```python
from build123d import *

# Parameters (mm, degrees)
SKETCH1_R           = 10
SKETCH1_R_2         = 2
SKETCH1_R_3         = 1.5
BOSS_EXTRUDE1_DEPTH = 2.3
SKETCH2_R           = 2.915
CUT_EXTRUDE1_DEPTH  = 1


with BuildPart() as part:
    # Sketch1 → Boss-Extrude1 (new body)
    with BuildSketch(Plane(origin=(0, 16.875, 0), x_dir=(1, 0, 0), z_dir=(0, 1, 0))):
        Circle(SKETCH1_R)
        Circle(SKETCH1_R_2, mode=Mode.SUBTRACT)
        with Locations((0, 6)):
            Circle(SKETCH1_R_3, mode=Mode.SUBTRACT)
        with Locations((0, -6)):
            Circle(SKETCH1_R_3, mode=Mode.SUBTRACT)
    extrude(amount=BOSS_EXTRUDE1_DEPTH)

    # Sketch2 → Cut-Extrude1 (cut)
    with BuildSketch(Plane(origin=(0, 19.175, 0), x_dir=(1, 0, 0), z_dir=(0, 1, 0))):
        with Locations((0, 6)):
            Circle(SKETCH2_R)
        with Locations((0, -6)):
            Circle(SKETCH2_R)
    extrude(amount=-CUT_EXTRUDE1_DEPTH, mode=Mode.SUBTRACT)


solid = part.part
```
Input: part model. Units: mm. Frame: model coordinates. A direction names the side the tool comes from. Coordinates: 2 decimals unless noted, no trailing zeros. Write each loop counter-clockwise with the first axis right and the second up, starting at its lowest first coordinate (ties: lowest second). Pieces come first, ordered by that corner, then holes.
1) Section A-A on z = 6. Output: boundary loops of the cut face in (x, y) (3 decimals).
2) Section D-D on z = 0. Output: boundary loops of the cut face in (x, y) (3 decimals), and give its area (3 significant figures).
3) Set-up query: faces 1 (the cylindrical face through (-0.325, 17.516, -4.536)), 2 (the flat face through (1.3, 18.175, -4.7)). Return all of +Z, -Z, +X, -X, +Y, -Y with unobstructed straight access to the full face (end or side cutting, diameter ignored); none if empty.
4) Material intervals for line 1 along Z through (x, y) = (0, 17.3); line 2 along Z through (x, y) = (0, 18.55) (3 decimals); line 3 along X through (y, z) = (18.3, 0), sorted ascending.
5) Pin query (flat end, axial travel): pin 1 Ø1 at (y, z) = (18.5, -4.5) entering from -X; pin 2 Ø2.5 at (x, z) = (0, 0) entering from +Y; pin 3 Ø1.7 at (x, z) = (1, -6) entering from +Y (3 decimals); pin 4 Ø7.5 at (x, z) = (0, -6) entering from -Y (3 decimals). Return the tip coordinate at first contact, or that it passes through.
6) Section B-B on x = 0. Output: boundary loops of the cut face in (y, z) (3 decimals).
7) Mould query, pull axis X, two halves, no side actions, for faces 3 (the cylindrical face through (-2.17, 18.01, 9.76)), 4 (the flat face through (1.3, 18.175, 7.3)), 5 (the flat face through (-2.4, 16.875, -0.1)). Classes: pulls with the +X half, pulls with the -X half, needs draft (parallel to the pull), parting line crosses it, or undercut.
8) Section C-C on y = 17.4. Output: boundary loops of the cut face in (x, z), and give its area (3 significant figures).
Check result:
1. outline: (-8, 16.875) - (-1.5, 16.875) - (-1.5, 18.175) - (-2.915, 18.175) - (-2.915, 19.175) - (-8, 19.175) - close; (1.5, 16.875) - (8, 16.875) - (8, 19.175) - (2.915, 19.175) - (2.915, 18.175) - (1.5, 18.175) - close
2. outline: (-10, 16.875) - (-2, 16.875) - (-2, 19.175) - (-10, 19.175) - close; (2, 16.875) - (10, 16.875) - (10, 19.175) - (2, 19.175) - close
2. area: 36.8 mm2
3. face 1: +Y, -Y
3. face 2: +Y
4. line 1: z = -10 to -7.5, -4.5 to -2, 2 to 4.5, 7.5 to 10
4. line 2: z = -10 to -8.915, -3.085 to -2, 2 to 3.085, 8.915 to 10
4. line 3: x = -10 to -2, 2 to 10
5. pin 1: stops at x = -9.17
5. pin 2: passes through
5. pin 3: stops at y = 18.175
5. pin 4: stops at y = 16.875
6. outline: (16.875, -10) - (19.175, -10) - (19.175, -8.915) - (18.175, -8.915) - (18.175, -7.5) - (16.875, -7.5) - close; (16.875, -4.5) - (18.175, -4.5) - (18.175, -3.085) - (19.175, -3.085) - (19.175, -2) - (16.875, -2) - close; (16.875, 2) - (19.175, 2) - (19.175, 3.085) - (18.175, 3.085) - (18.175, 4.5) - (16.875, 4.5) - close; (16.875, 7.5) - (18.175, 7.5) - (18.175, 8.915) - (19.175, 8.915) - (19.175, 10) - (16.875, 10) - close
7. face 3: parting line crosses it
7. face 4: undercut
7. face 5: needs draft
8. outline: circle Ø20 at (0, 0); hole circle Ø4 at (0, 0); hole circle Ø3 at (0, -6); hole circle Ø3 at (0, 6)
8. area: 287 mm2
